Source: CAD feature listing. Evaluate the final solid. Frame: model axes, mm. A direction names the side the tool comes from. Coordinates: 2 decimals unless noted, no trailing zeros. Write each loop counter-clockwise with the first axis right and the second up, starting at its lowest first coordinate (ties: lowest second). Pieces come first, ordered by that corner, then holes. Notation, with made-up numbers: M -7,30.5 L 17,30.5 A19 ccw 17,47.5 Z; hole C -20.5,41.25 d9. An arc over 180 degrees is marked long. One line per item, written item: value. Start each with the question number.
Item 1: Cut plane C-C, the plane z = 16. Output: boundary loops of the cut face in (x, y) (3 decimals).
Item 2: Cut plane D-D, the plane x = 2.75. Output: boundary loops of the cut face in (y, z), then the cut area to 3 significant figures.
Item 3: Ray query, L1, parallel to Z at x = 4.75, y = -0.5; L2, parallel to X at y = 0, z = 18.5 (3 decimals); L3, parallel to Y at x = 3.5, z = 11. Return the intervals inside material, ascending. Write a range as from..to.
Item 4: Cut plane A-A, the plane x = 0. Output: boundary loops of the cut face in (y, z) (3 decimals).
Item 5: Pin query (flat end, axial travel): P1, Ø0.6, axis at x = 5, y = -0.5, coming from the +Z side; P2, Ø0.8, axis at x = -5, y = 0.5, coming from the +Z side; P3, Ø1.2, axis at x = -4.5, z = 30, coming from the +Y side. Return the tip coordinate at first contact, or that it passes through.
Item 6: Set-up query: faces 1 (the flat face through (-0.833, 4, 26)), 2 (the flat face through (3, 3, 31.5)), 3 (the flat face through (0, 4.5, 24)), 4 (the flat face through (-5.333, 0, 31)), 5 (the flat face through (0, 1, 42)). Return all of +Z, -Z, +X, -X, +Y, -Y with unobstructed straight access to the full face (end or side cutting, diameter ignored); none if empty.
Item 7: Cut plane B-B, the plane y = 1.5. Output: boundary loops of the cut face in (x, z), then the cut area to 3 significant figures.
```python
from build123d import *

# Parameters (mm, degrees)
BOSS_EXTRUDE1_DEPTH      = 42
BOSS_EXTRUDE2_START      = -5
BOSS_EXTRUDE2_DEPTH      = 5.5
BOSS_EXTRUDE4_DEPTH      = 2.5
BOSS_EXTRUDE4_DEPTH_BACK = 3
SKETCH6_W                = 1.666666666
SKETCH6_H                = 4.236096709
BOSS_EXTRUDE5_DEPTH      = 10


with BuildPart() as part:
    # Sketch1 → Boss-Extrude1 (new body)
    with BuildSketch(Plane.XY):
        with BuildLine():
            Line((3.829096611, -0.815625), (-3.829096611, -0.815625))
            ThreePointArc((-3.829096611, -0.815625), (0, 3.915), (3.829096611, -0.815625))
        make_face()
    extrude(amount=BOSS_EXTRUDE1_DEPTH)

    # Sketch2 → Boss-Extrude2 (add)
    with BuildSketch(Plane.XY.offset(42).offset(BOSS_EXTRUDE2_START)):
        with BuildLine():
            Line((4.594837716, -0.815625), (-4.594837716, -0.815625))
            ThreePointArc((-4.594837716, -0.815625), (-4.648674746, -0.40939087), (-4.666666667, 0))
            ThreePointArc((-4.666666667, 0), (0, 4.666666667), (4.666666667, 0))
            ThreePointArc((4.666666667, 0), (4.648674746, -0.40939087), (4.594837716, -0.815625))
        make_face()
    extrude(amount=-BOSS_EXTRUDE2_DEPTH)

    # Sketch5 → Boss-Extrude4 (add, two sides: drawn at the far end of the back side and taken through both)
    with BuildSketch(Plane.XY.offset(31.5).offset(-BOSS_EXTRUDE4_DEPTH_BACK)):
        with BuildLine():
            Line((5.333333333, 0.833333333), (3.825281762, 0.833333333))
            ThreePointArc((3.825281762, 0.833333333), (2.768323048, 2.768323048), (0.833333333, 3.825281762))
            Line((0.833333333, 3.825281762), (0.833333333, 5.333333333))
            Line((0.833333333, 5.333333333), (-0.833333333, 5.333333333))
            Line((-0.833333333, 5.333333333), (-0.833333333, 3.825281762))
            ThreePointArc((-0.833333333, 3.825281762), (-2.768323048, 2.768323048), (-3.825281762, 0.833333333))
            Line((-3.825281762, 0.833333333), (-5.333333333, 0.833333333))
            Line((-5.333333333, 0.833333333), (-5.333333333, -0.815625))
            Line((-5.333333333, -0.815625), (5.333333333, -0.815625))
            Line((5.333333333, -0.815625), (5.333333333, 0.833333333))
        make_face()
    extrude(amount=BOSS_EXTRUDE4_DEPTH + BOSS_EXTRUDE4_DEPTH_BACK)

    # Sketch6 → Boss-Extrude5 (add)
    with BuildSketch(Plane(origin=(0, 0, 28.5), x_dir=(-1, 0, 0), z_dir=(0, 0, -1))):
        with Locations((0, 2.381951646)):
            Rectangle(SKETCH6_W, SKETCH6_H)
    extrude(amount=BOSS_EXTRUDE5_DEPTH)


solid = part.part
```
From the geometry:
1. outline: M -3.829,-0.816 L 3.829,-0.816 A3.915 ccw long Z
2. outline: M -0.82,0 L 2.79,0 L 2.79,31.5 L 3.77,31.5 L 3.77,37 L 2.79,37 L 2.79,42 L -0.82,42 Z
2. area: 157 mm²
3. L1: z = 28.5..34
3. L2: x = -3.915..3.915
3. L3: y = -0.82..1.75
4. outline: M -0.816,0 L 3.915,0 L 3.915,18.5 L 4.5,18.5 L 4.5,28.5 L 5.333,28.5 L 5.333,34 L 4.667,34 L 4.667,37 L 3.915,37 L 3.915,42 L -0.816,42 Z
5. P1: stops at z = 34
5. P2: stops at z = 37
5. P3: stops at y = 0.83
6. face 1: -Z, -X, +Y
6. face 2: -Z, +X, +Y
6. face 3: -Z, +X, -X, +Y
6. face 4: +Z, -Z, -X, +Y, -Y
6. face 5: +Z, +X, -X, +Y, -Y
7. outline: M -4.42,31.5 L -3.62,31.5 L -3.62,0 L 3.62,0 L 3.62,31.5 L 4.42,31.5 L 4.42,37 L 3.62,37 L 3.62,42 L -3.62,42 L -3.62,37 L -4.42,37 Z
7. area: 313 mm²
